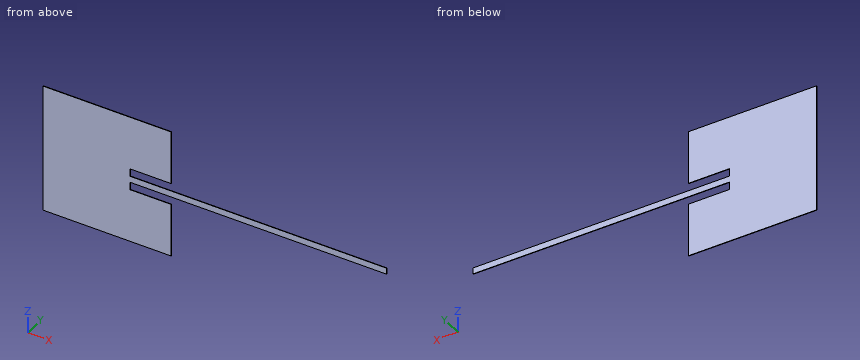
Autodesk Inventor part; units mm, degrees
ref_plane "YZ Plane" through (0, 0, 0) normal (1, 0, 0) x (0, 1, 0)
ref_plane "XZ Plane" through (0, 0, 0) normal (0, 1, 0) x (-1, 0, 0)
ref_plane "XY Plane" through (0, 0, 0) normal (0, 0, 1) x (1, 0, 0)
sketch "Sketch1" plane through (0, 0, 0) normal (0, 1, 0) x (-1, 0, 0)
  line L0 (0, 0) -> (0, 0.6)
  line L1 (0, 0.6) -> (50, 0.6)
  line L2 (50, 0.6) -> (50, 2.1)
  line L3 (50, 2.1) -> (42, 2.1)
  line L4 (42, 2.1) -> (42, 12.5)
  line L5 (42, 12.5) -> (67, 12.5)
  line L6 (67, 12.5) -> (67, 0)
  line L7 (67, 0) -> (0, 0)
  line L8 (0, 0) -> (0, -0.6)
  line L9 (0, -0.6) -> (50, -0.6)
  line L10 (50, -0.6) -> (50, -2.1)
  line L11 (50, -2.1) -> (42, -2.1)
  line L12 (42, -2.1) -> (42, -12.5)
  line L13 (42, -12.5) -> (67, -12.5)
  line L14 (67, -12.5) -> (67, 0)
  dimension "d1" = 0.6
  dimension "d2" = 50
  dimension "d3" = 1.5
  dimension "d4" = 12.5
  dimension "d5" = 25
  dimension "d6" = 8
extrude "Extrusion1" add sketch "Sketch1" along normal blind 0.1
Geometry check sheet. Reference: the model listing, model coordinates, mm. Coordinates: 2 decimals unless noted, no trailing zeros. Loops run counter-clockwise (first coordinate to the right, second up) from the corner with the lowest first, then second, coordinate; pieces in that order, holes last. Notation, with made-up numbers: (86.25, 51.5) -> (121.25, 51.5) arc R9 cw to (121.25, 58.5) -> close; hole circle Ø6 at (25, 38.5). An arc over 180 degrees is marked (long way). Put each result on its own line as item: value.
1) Cross-section at C-C on z = 6.75. Record the boundary of the cut face in (x, y).
Result set:
outline: (-67, 0) -> (-42, 0) -> (-42, 0.1) -> (-67, 0.1) -> close
2) Cross-section at A-A on x = -47. Record the boundary of the cut face in (y, z).
Result set:
outline: (0, -12.5) -> (0.1, -12.5) -> (0.1, -2.1) -> (0, -2.1) -> close; (0, -0.6) -> (0.1, -0.6) -> (0.1, 0.6) -> (0, 0.6) -> close; (0, 2.1) -> (0.1, 2.1) -> (0.1, 12.5) -> (0, 12.5) -> close
3) Cross-section at D-D on x = -28. Record the boundary of the cut face in (y, z).
Result set:
outline: (0, -0.6) -> (0.1, -0.6) -> (0.1, 0.6) -> (0, 0.6) -> close
4) Gauge pin test, flat end, axial feed: pin 1 Ø5 at (x, z) = (-30.5, -3) entering from -Y. Record the tip position at first contact, or that the pin passes through.
Result set:
pin 1: stops at y = 0
5) Thickness scan on line 1 (Z direction, x = -46.5, y = 0.05); line 2 (Z direction, x = -26.5, y = 0.05). Record the ranges inside material, lowest first.
Result set:
line 1: z = -12.5 to -2.1, -0.6 to 0.6, 2.1 to 12.5
line 2: z = -0.6 to 0.6
6) Cross-section at B-B on y = 0.05. Record the boundary of the cut face in (x, z), plus the area to 3 significant figures.
Result set:
outline: (-67, -12.5) -> (-42, -12.5) -> (-42, -2.1) -> (-50, -2.1) -> (-50, -0.6) -> (0, -0.6) -> (0, 0.6) -> (-50, 0.6) -> (-50, 2.1) -> (-42, 2.1) -> (-42, 12.5) -> (-67, 12.5) -> close
area: 651 mm^2
